Can you work these out from the model? Positions are in its coordinate system, mm. A direction names the side the tool comes from. Coordinates: 2 decimals unless noted, no trailing zeros. Loops run counter-clockwise (first coordinate to the right, second up) from the corner with the lowest first, then second, coordinate; pieces in that order, holes last. Notation, with made-up numbers: M 68.25,-24 L 90.25,-24 A15 ccw 90.25,-9 Z; hole C 38,-31.5 d9. An arc over 180 degrees is marked long. Return JSON: item names as keys, results as strings. Group by question number.
```python
from build123d import *

# Parameters (mm, degrees)
BOSS_EXTRUDE1_DEPTH = 35
SKETCH2_W           = 35
SKETCH2_H           = 55
BOSS_EXTRUDE2_DEPTH = 83.45
BOSS_EXTRUDE3_DEPTH = 20
SKETCH4_W           = 122.95
SKETCH4_H           = 15
BOSS_EXTRUDE4_DEPTH = 55
SKETCH5_R           = 73
CUT_EXTRUDE1_DEPTH  = 3.5
CUT_EXTRUDE2_REACH  = 221.708
SKETCH6_R           = 40


with BuildPart() as part:
    # Sketch1 → Boss-Extrude1 (new body)
    with BuildSketch(Plane.XY):
        with BuildLine():
            Line((-95, -77), (-87.95, -77))
            Line((-87.95, -77), (-87.95, -95))
            Line((-87.95, -95), (-87.95, -117))
            Line((-87.95, -117), (95, -117))
            Line((95, -117), (95, -95))
            Line((95, -95), (95, 0))
            ThreePointArc((95, 0), (16.050772972, 93.63424954), (-89.576267094, 31.640043828))
            Line((-89.576267094, 31.640043828), (-127.95, -77))
            Line((-127.95, -77), (-95, -77))
        make_face()
    extrude(amount=BOSS_EXTRUDE1_DEPTH)

    # Sketch2 → Boss-Extrude2 (add)
    with BuildSketch(Plane(origin=(0, 0, 0), x_dir=(-1, 0, 0), z_dir=(0, 0, -1))):
        Polygon((127.95, -77), (122.651714273, -62), (88.977103652, -62), (62.95, -62), (62.95, -117), (87.95, -117), (87.95, -77), align=None)
        with Locations((-77.5, -89.5)):
            Rectangle(SKETCH2_W, SKETCH2_H)
    extrude(amount=BOSS_EXTRUDE2_DEPTH)

    # Sketch3 → Boss-Extrude3 (add)
    with BuildSketch(Plane(origin=(0, 0, -83.45), x_dir=(-1, 0, 0), z_dir=(0, 0, -1))):
        Polygon((127.95, -77), (-95, -77), (-95, -62), (122.651714273, -62), align=None)
    extrude(amount=BOSS_EXTRUDE3_DEPTH)

    # Sketch4 → Boss-Extrude4 (add)
    with BuildSketch(Plane(origin=(0, -62, 0), x_dir=(1, 0, 0), z_dir=(0, 1, 0))):
        with Locations((-1.475, 75.95)):
            Rectangle(SKETCH4_W, SKETCH4_H)
    extrude(amount=-BOSS_EXTRUDE4_DEPTH)

    # Sketch5 → Cut-Extrude1 (cut)
    with BuildSketch(Plane.XY.offset(35)):
        Circle(SKETCH5_R)
    extrude(amount=-CUT_EXTRUDE1_DEPTH, mode=Mode.SUBTRACT)

    # Sketch6 → Cut-Extrude2 (cut, up to next)
    with BuildSketch(Plane.XY.offset(31.5), mode=Mode.PRIVATE) as cut_extrude2_sk1:
        Circle(SKETCH6_R)
    cut_extrude2_tool1 = extrude(cut_extrude2_sk1.sketch, amount=-CUT_EXTRUDE2_REACH, mode=Mode.PRIVATE) & part.part
    add(cut_extrude2_tool1.solids().sort_by_distance((0, 0, 31.5))[0], mode=Mode.SUBTRACT)


solid = part.part
```
1) If I drill on line 1 (Z direction, x = -62, y = -62.5); line 2 (Y direction, x = 0, z = 32.75); line 3 (Y direction, x = 78.5, z = -69.5), over which ranges is the centre line in solid material (lowest first)? Write a range as from..to.
2) For faces 1 (the face through (-87.95, -97, -23)), 2 (the face through (-15.825, -71.264, 33.274)), 3 (the face through (-40, -10, 0)), which set-ups out of +Z, -Z, +X, -X, +Y, -Y let a thin tool reach every point of the face, with its end or its side?
3) Suppose I cut it at B-B, the plane x = 0. List the corners of the cut face in (y, z) for me, then the cut area to 3 significant figures.
4) Suppose I cut it at C-C, the plane z = 15.5. List the corners of the cut face in (x, y) for me.
5) Suppose I cut it at D-D, the plane y = -37. List the corners of the cut face in (x, z) for me.
6) Suppose I cut it at A-A, the plane z = -33. List the corners of the cut face in (x, y) for me.
7) For pin 1 (20 mm diameter, centred on x = -12, y = -97, fed in from -Z); pin 2 (12 mm diameter, centred on y = -100.5, z = -5, fed in from -X), each with a flat end and sliding along its axis, tell me the tip position at first contact or that it passes through.
8) If we mould it in two halves opening along X, with no side actions, what happens to faces 4 (the face through (31, -31, 31.5)), 5 (the face through (95, -72, -18)), 6 (the face through (2, -97, -83.45))? For each: +X half, -X half, draft (parallel to the pull), parting line (faces both ways), or undercut.
Returned:
{
 "1": {"line 1": "z = -103.45..-68.45, 0..35", "line 2": "y = -117..-73, 73..95", "line 3": "y = -117..-62"},
 "2": {"face 1": "+Z, -Z, -X, -Y", "face 2": "+Z", "face 3": "+Y"},
 "3": {"outline": "M -117,-83.45 L -77,-83.45 L -77,-103.45 L -62,-103.45 L -62,-68.45 L -117,-68.45 Z; M -117,0 L -40,0 L -40,31.5 L -73,31.5 L -73,35 L -117,35 Z; M 40,0 L 95,0 L 95,35 L 73,35 L 73,31.5 L 40,31.5 Z", "area": "5,510 mm²"},
 "4": {"outline": "M -127.95,-77 L -87.95,-77 L -87.95,-117 L 95,-117 L 95,0 A95 ccw -89.58,31.64 Z; hole C 0,0 d80"},
 "5": {"outline": "M -113.82,0 L -15.2,0 L -15.2,31.5 L -62.93,31.5 L -62.93,35 L -113.82,35 Z; M 15.2,0 L 95,0 L 95,35 L 62.93,35 L 62.93,31.5 L 15.2,31.5 Z"},
 "6": {"outline": "M -127.95,-77 L -87.95,-77 L -87.95,-117 L -62.95,-117 L -62.95,-62 L -122.65,-62 Z; M 60,-117 L 95,-117 L 95,-62 L 60,-62 Z"},
 "7": {"pin 1": "stops at z = -83.45", "pin 2": "stops at x = -87.95"},
 "8": {"face 4": "undercut", "face 5": "+X half", "face 6": "draft"}
}
